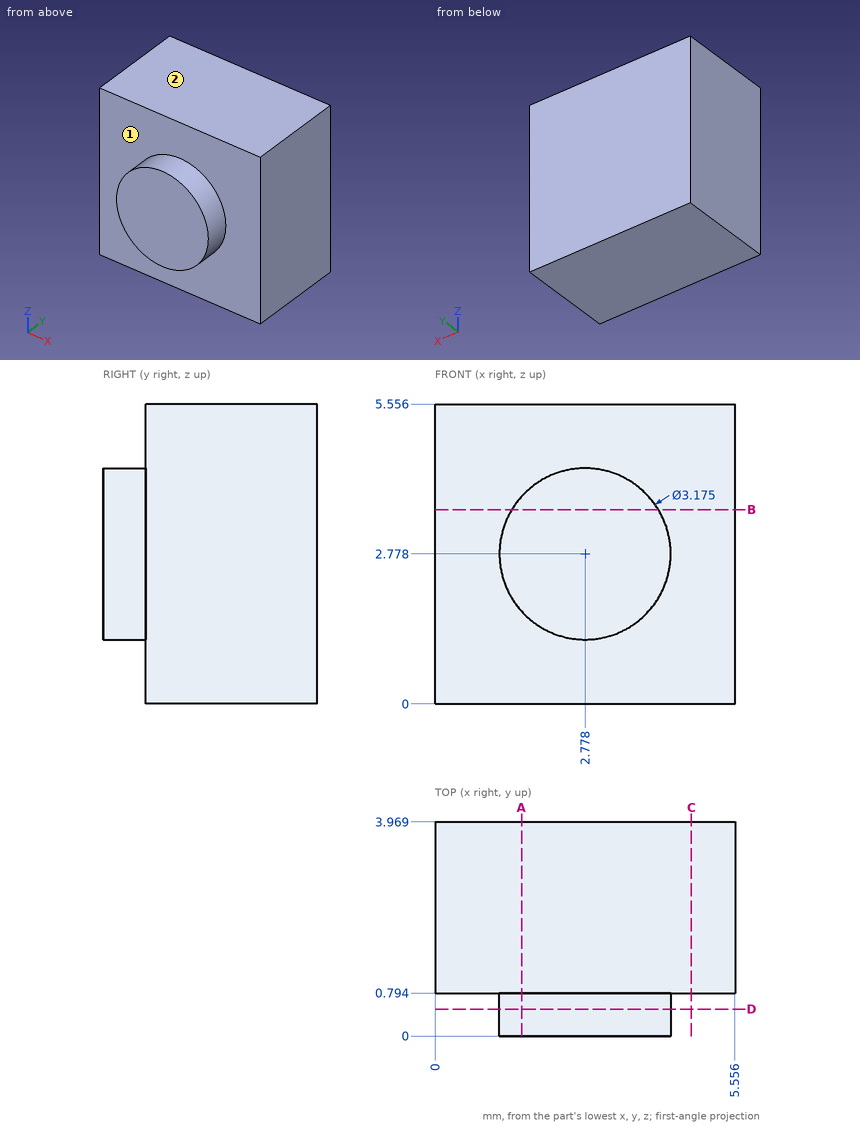
Here's the drawing with two shaded views (mm, measured from the low corner). I have some questions. A direction names the side the tool comes from. Give positions to 0.01 mm unless a question says otherwise; leave off trailing zeros. Order: outer loops, then holes, each group sorted by start corner. A loop starts at its lowest first (then second) coordinate and runs counter-clockwise, first axis right, second up. Notation, with made-up numbers: (-9.5, -27.75) - (15.5, -27.75) arc R26 ccw to (15.5, 4.25) - close; hole circle Ø1 at (13.25, -17.5). An arc over 180 degrees is marked (long way). Use a Markdown table: item, result. Add a question column.
Q1. On a 3-axis mill with a long thin cutter (end or side, diameter ignored), from which of +Z, -Z, +X, -X, +Y, -Y can I reach the whole of each face in a straight line? I mean the marked faces 1 and 2. Say none if no direction works.
Q2. If we section it at D-D on y = 0.5: Write out the boundary of the cut face in (x, z) (1 decimal).
Q3. If we section it at B-B on z = 3.6: Write out the boundary of the cut face in (x, y).
Q4. If we section it at A-A on x = 1.6: Write out the boundary of the cut face in (y, z), plus the area to 3 significant figures.
Q5. Please list where these lines run through material, in increasing order: line 1 along Y through (x, z) = (4.4, 4.8); line 2 along X through (y, z) = (0.4, 3.4).
Q6. If we section it at C-C on x = 4.75: Write out the boundary of the cut face in (y, z).
Answers follow:
| question | item | result |
|---|---|---|
| 1 | face 1 | -Y |
| 1 | face 2 | +Z, +X, -X, +Y, -Y |
| 2 | outline | circle Ø3.2 at (2.8, 2.8) |
| 3 | outline | (0, 0.79) - (1.42, 0.79) - (1.42, 0) - (4.14, 0) - (4.14, 0.79) - (5.56, 0.79) - (5.56, 3.97) - (0, 3.97) - close |
| 4 | outline | (0, 1.71) - (0.79, 1.71) - (0.79, 0) - (3.97, 0) - (3.97, 5.56) - (0.79, 5.56) - (0.79, 3.84) - (0, 3.84) - close |
| 4 | area | 19.3 mm^2 |
| 5 | line 1 | y = 0.79 to 3.97 |
| 5 | line 2 | x = 1.32 to 4.24 |
| 6 | outline | (0.79, 0) - (3.97, 0) - (3.97, 5.56) - (0.79, 5.56) - close |
